Could you check a few things on this drawing? It's one solid part, dimensions in mm from its lowest x, y, z. Give positions to 0.01 mm unless a question says otherwise; leave off trailing zeros. Order: outer loops, then holes, each group sorted by start corner. A loop starts at its lowest first (then second) coordinate and runs counter-clockwise, first axis right, second up. Notation, with made-up numbers: M 20.25,-4 L 51.25,-4 A14 ccw 51.25,17 Z; hole C -30,4 d7. An arc over 180 degrees is marked long. Use one line per item in the form item = value.
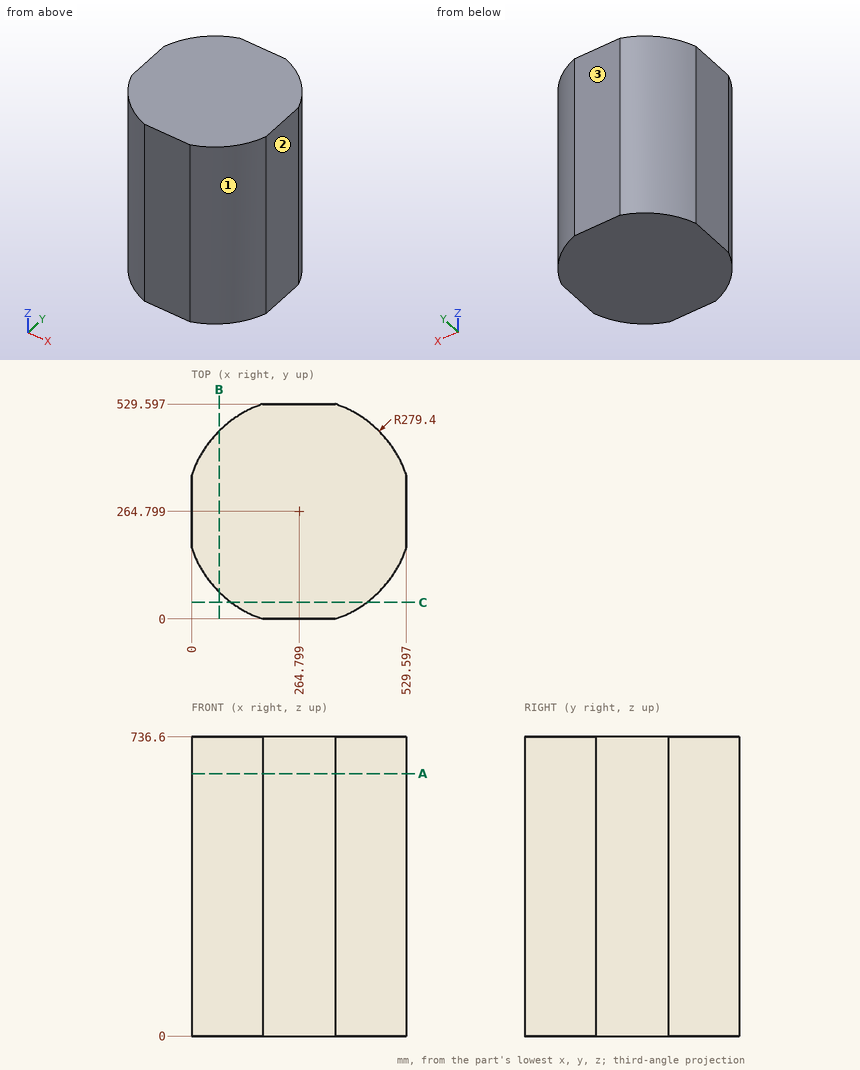
Q1. I need wall thicknesses on L1, parallel to X at y = 78.5, z = 257 (1 decimal); L2, parallel to Y at x = 438, z = 285 (1 decimal); L3, parallel to Y at x = 390, z = 615 (1 decimal). Which ranges of each line are inside material? Lowest first, please.
Found:
L1 = 56.6 to 473
L2 = 45.6 to 484
L3 = 15 to 514.6
Q2. I want a section at A-A on z = 646.5. Write out the boundary of the cut face in (x, y).
Found:
outline = M 0,175.66 A279.4 ccw 175.66,0 L 353.94,0 A279.4 ccw 529.6,175.66 L 529.6,353.94 A279.4 ccw 353.94,529.6 L 175.66,529.6 A279.4 ccw 0,353.94 Z
Q3. Thinking about a two-plate mould opening in Y: for the marked faces 1, 2 and 3, which applies, +Y half, -Y half, draft (parallel to the pull), parting line (faces both ways), or undercut?
Found:
face_1 = -Y half
face_2 = draft
face_3 = +Y half
Q4. I want a section at C-C on y = 41. Write out the boundary of the cut face in (x, z), then the cut area to 3 significant figures.
Found:
outline = M 97.53,0 L 432.07,0 L 432.07,736.6 L 97.53,736.6 Z
area = 246,000 mm²
Q5. I want a section at B-B on x = 68. Write out the boundary of the cut face in (y, z).
Found:
outline = M 66.47,0 L 463.13,0 L 463.13,736.6 L 66.47,736.6 Z
Q6. I'm going to push flat-ended pins straight in: pin 1 Ø8 at (x, z) = (170, 577) entering from +Y; pin 2 Ø10 at (y, z) = (126.5, 616) entering from -X; pin 3 Ø1 at (x, z) = (159.5, 460) entering from -Y. Where does each tip first touch, or does it pass through?
Found:
pin_1 = 529.03
pin_2 = 19.25
pin_3 = 5.8
